Geometry: final body of the model. Coordinates: model frame, mm. A direction names the side the tool comes from. Round coordinates to 2 decimals unless told otherwise and drop trailing zeros. Loops run counter-clockwise (first coordinate to the right, second up) from the corner with the lowest first, then second, coordinate; pieces in that order, holes last. Notation, with made-up numbers: (27, -0.5) - (51, -0.5) arc R22 cw to (51, 38.5) - close; hole circle Ø3 at (2, 16). An arc over 180 degrees is marked (long way). Answer in a Markdown table with one row per item. Add a question column.
from build123d import *

# Parameters (mm, degrees)
SKETCH_2_R          = 1.6
CUT_EXTRUDE_1_DEPTH = 10
EXTRUDE_START       = -28
EXTRUDE_1_DEPTH     = 28
HOLE_WIZARD_M3_2_D  = 2.5


with BuildPart() as part:
    # 草图1 → 旋转1 (revolve)
    with BuildSketch(Plane.XY, mode=Mode.PRIVATE) as revolve_1_sk:
        Polygon((-5.25, 0), (-18, 0), (-18, 3), (-8, 3), (-8, 28), (-5.25, 28), align=None)
    revolve(revolve_1_sk.sketch.rotate(Axis((0, 12.843932511, 0), (0, -1, 0)), 270), axis=Axis((0, 12.843932511, 0), (0, -1, 0)))

    # 草图2 → 切除-拉伸1 (cut)
    with BuildSketch(Plane(origin=(0, 3, 0), x_dir=(1, 0, 0), z_dir=(0, 1, 0))):
        with Locations(Location((0, 14, 0), (0, 0, 270))):
            Circle(SKETCH_2_R)
        with Locations(Location((12.124355653, 7, 0), (0, 0, 270))):
            Circle(SKETCH_2_R)
        with Locations(Location((12.124355653, -7, 0), (0, 0, 270))):
            Circle(SKETCH_2_R)
        with Locations(Location((0, -14, 0), (0, 0, 270))):
            Circle(SKETCH_2_R)
        with Locations(Location((-12.124355653, -7, 0), (0, 0, 270))):
            Circle(SKETCH_2_R)
        with Locations(Location((-12.124355653, 7, 0), (0, 0, 270))):
            Circle(SKETCH_2_R)
    extrude(amount=-CUT_EXTRUDE_1_DEPTH, mode=Mode.SUBTRACT)

    # 草图3 → 凸台-拉伸1 (add)
    with BuildSketch(Plane(origin=(0, 28, 0), x_dir=(1, 0, 0), z_dir=(0, 1, 0)).offset(EXTRUDE_START)):
        with BuildLine():
            Line((-3.082207001, 4.25), (3.082207001, 4.25))
            ThreePointArc((3.082207001, 4.25), (0, 5.25), (-3.082207001, 4.25))
        make_face()
    extrude(amount=EXTRUDE_1_DEPTH)

    # M3 螺纹孔2 (through all)
    with Locations(Plane(origin=(0, 0, -10), x_dir=(1, 0, 0), z_dir=(0, 0, -1))):
        with Locations((0, -22)):
            Hole(HOLE_WIZARD_M3_2_D / 2)


solid = part.part
1) Section D-D, the plane y = 22. Return the cut outline in (x, z).
2) Section B-B, the plane z = 0. Return the cut outline in (x, y), and give its area (3 significant figures).
3) Pull-direction query (Y, two-part tool) for faces 1 (the cylindrical face through (0.27, 23.22, 6.57)), 2 (the cylindrical face through (0.07, 1.52, 12.4)), 3 (the flat face through (4, 3, 8)); classes: pulls with the +Y half, pulls with the -Y half, needs draft (parallel to the pull), parting line crosses it, or undercut.
4) Reachability of faces 4 (the cylindrical face through (0.27, 23.22, -6.1)), 5 (the flat face through (0, 14, -4.25)), 6 (the cylindrical face through (3.06, 15.68, 7.39)) from +Z, -Z, +X, -X, +Y, -Y: full face, straight path, thin tool, end or side. Return the list, or none.
5) Contact query for flat-ended pins moving along their axis: pin 1 Ø4 at (x, y) = (2, 4.5) entering from +Z; pin 2 Ø3 at (x, y) = (0, 22) entering from +Z; pin 3 Ø12 at (x, z) = (-9, 10) entering from +Y; pin 4 Ø2 at (y, z) = (3.5, -1.5) entering from -X. Output: stop coordinate, or through.
6) Section A-A, the plane z = 6. Return the cut outline in (x, y).
7) Section C-C, the plane x = -0.5. Return the cut outline in (y, z), and give its area (3 significant figures).
8) Material intervals for line 1 along X through (y, z) = (1.55, -7); line 2 along Y through (x, z) = (-14, 3); line 3 along X through (y, z) = (17, -4), sorted ascending. Write a range as from..to.
Evaluation:
| question | item | result |
|---|---|---|
| 1 | outline | (-3.08, -4.25) arc R5.25 cw to (-1.25, 5.1) - (-1.25, 7.9) arc R8 ccw to (-1.25, -7.9) - (-1.25, -4.25) - close; (1.25, -7.9) arc R8 ccw to (1.25, 7.9) - (1.25, 5.1) arc R5.25 cw to (3.08, -4.25) - (1.25, -4.25) - close |
| 2 | outline | (-18, 0) - (-5.25, 0) - (-5.25, 28) - (-8, 28) - (-8, 3) - (-18, 3) - close; (5.25, 0) - (18, 0) - (18, 3) - (8, 3) - (8, 28) - (5.25, 28) - close |
| 2 | area | 214 mm² |
| 3 | face 1 | undercut |
| 3 | face 2 | needs draft |
| 3 | face 3 | pulls with the +Y half |
| 4 | face 4 | +Z, -Z |
| 4 | face 5 | +Y, -Y |
| 4 | face 6 | +Y |
| 5 | pin 1 | stops at z = 17.99 |
| 5 | pin 2 | stops at z = 8 |
| 5 | pin 3 | stops at y = 28 |
| 5 | pin 4 | stops at x = -17.99 |
| 6 | outline | (-16.97, 0) - (-13.37, 0) - (-13.37, 3) - (-16.97, 3) - close; (-10.88, 0) - (10.88, 0) - (10.88, 3) - (5.29, 3) - (5.29, 28) - (-5.29, 28) - (-5.29, 3) - (-10.88, 3) - close; (13.37, 0) - (16.97, 0) - (16.97, 3) - (13.37, 3) - close; hole circle Ø2.5 at (0, 22) |
| 7 | outline | (0, -17.99) - (3, -17.99) - (3, -15.52) - (0, -15.52) - close; (0, -12.48) - (3, -12.48) - (3, -7.98) - (20.85, -7.98) - (20.85, -4.25) - (0, -4.25) - close; (0, 5.23) - (20.85, 5.23) - (20.85, 7.98) - (3, 7.98) - (3, 12.48) - (0, 12.48) - close; (0, 15.52) - (3, 15.52) - (3, 17.99) - (0, 17.99) - close; (23.15, -7.98) - (28, -7.98) - (28, -4.25) - (23.15, -4.25) - close; (23.15, 5.23) - (28, 5.23) - (28, 7.98) - (23.15, 7.98) - close |
| 7 | area | 209 mm² |
| 8 | line 1 | x = -16.58..-13.72, -10.52..10.52, 13.72..16.58 |
| 8 | line 2 | y = 0..3 |
| 8 | line 3 | x = -6.93..-3.4, 3.4..6.93 |
